from build123d import *

# Parameters (mm, degrees)
SM_BASE_FLANGE_1_DEPTH   = 61.75
SKETCH_3_R               = 25
CUT_EXTRUDE_1_DEPTH      = 4
EXTRUDE_2_DEPTH          = 4
CUT_EXTRUDE_3_DEPTH      = 4
SM_START                 = -122
SM_EDGE_FLANGE_1_DEPTH   = 244
SM_EDGE_FLANGE_1_2_DEPTH = 33
SM_START_2               = 89
SM_EDGE_FLANGE_1_3_DEPTH = 33
SKETCH_44_R              = 3.25
CUT_EXTRUDE_4_DEPTH      = 4
CHAMFER_1_SIZE           = 4


# Read off the part's stored shape, not the designer's step: Ребро-кромка1
# Sheet-metal steps are written as plain solids
with BuildPart() as part:
    # Sketch 1 → Базовая кромка1 (new, symmetric)
    with BuildSketch(Plane.XY):
        with BuildLine():
            Line((-67.211573407, -134), (-53.127605882, 0))
            Line((-53.127605882, 0), (-50.876471404, 21.418113853))
            ThreePointArc((-50.876471404, 21.418113853), (-49.574906248, 23.972579302), (-46.898383823, 25))
            Line((-46.898383823, 25), (46.898383823, 25))
            ThreePointArc((46.898383823, 25), (49.574906248, 23.972579302), (50.876471404, 21.418113853))
            Line((50.876471404, 21.418113853), (53.127605882, 0))
            Line((53.127605882, 0), (67.211573407, -134))
            Line((67.211573407, -134), (71.189660989, -133.581886147))
            Line((71.189660989, -133.581886147), (57.105693463, 0.418113853))
            Line((57.105693463, 0.418113853), (54.854558986, 21.836227706))
            ThreePointArc((54.854558986, 21.836227706), (52.251428674, 26.945158604), (46.898383823, 29))
            Line((46.898383823, 29), (-46.898383823, 29))
            ThreePointArc((-46.898383823, 29), (-52.251428674, 26.945158604), (-54.854558986, 21.836227706))
            Line((-54.854558986, 21.836227706), (-57.105693463, 0.418113853))
            Line((-57.105693463, 0.418113853), (-71.189660989, -133.581886147))
            Line((-71.189660989, -133.581886147), (-67.211573407, -134))
        make_face()
    extrude(amount=SM_BASE_FLANGE_1_DEPTH, both=True)

    # Эскиз3 → Вытянуть1 (cut)
    with BuildSketch(Plane(origin=(0, 29, 0), x_dir=(1, 0, 0), z_dir=(0, 1, 0))):
        with Locations(Location((0, 0, 0), (0, 0, 180))):
            Circle(SKETCH_3_R)
    extrude(amount=-CUT_EXTRUDE_1_DEPTH, mode=Mode.SUBTRACT)

    # Эскиз33 → Вытянуть2 (add)
    with BuildSketch(Plane(origin=(56.525210635, 5.941039037, 0), x_dir=(0, 0, -1), z_dir=(0.9945218953682734, 0.10452846326765315, 0))):
        with BuildLine():
            Line((-62.05448187, 13.177809809), (-121.69551813, -130.808388804))
            ThreePointArc((-121.69551813, -130.808388804), (-121.923141122, -131.558761245), (-122, -132.339122533))
            Line((-122, -132.339122533), (-122, -140.291456461))
            Line((-122, -140.291456461), (-61.75, -140.291456461))
            Line((-61.75, -140.291456461), (-61.75, 14.708543539))
            ThreePointArc((-61.75, 14.708543539), (-61.826858878, 13.928182251), (-62.05448187, 13.177809809))
        make_face()
        with BuildLine():
            Line((122, -132.339122533), (122, -140.291456461))
            Line((122, -140.291456461), (61.75, -140.291456461))
            Line((61.75, -140.291456461), (61.75, 14.708543539))
            ThreePointArc((61.75, 14.708543539), (61.826858878, 13.928182251), (62.05448187, 13.177809809))
            Line((62.05448187, 13.177809809), (121.69551813, -130.808388804))
            ThreePointArc((121.69551813, -130.808388804), (121.923141122, -131.558761245), (122, -132.339122533))
        make_face()
    extrude_2 = extrude(amount=-EXTRUDE_2_DEPTH)

    # Эскиз39 → Вытянуть3 (cut)
    with BuildSketch(Plane(origin=(56.525210635, 5.941039037, 0), x_dir=(0, 0, -1), z_dir=(0.9945218953682734, 0.10452846326765315, 0))):
        with BuildLine():
            Line((25.655356237, -12.291456461), (-25.655356237, -12.291456461))
            ThreePointArc((-25.655356237, -12.291456461), (-27.73044927, -12.871808979), (-29.20339957, -14.444462008))
            Line((-29.20339957, -14.444462008), (-88.548043333, -128.444462008))
            ThreePointArc((-88.548043333, -128.444462008), (-88.885368279, -129.340712892), (-89, -130.291456461))
            Line((-89, -130.291456461), (-89, -140.291456461))
            Line((-89, -140.291456461), (89, -140.291456461))
            Line((89, -140.291456461), (89, -130.291456461))
            ThreePointArc((89, -130.291456461), (88.885368279, -129.340712892), (88.548043333, -128.444462008))
            Line((88.548043333, -128.444462008), (29.20339957, -14.444462008))
            ThreePointArc((29.20339957, -14.444462008), (27.73044927, -12.871808979), (25.655356237, -12.291456461))
        make_face()
    cut_extrude_3 = extrude(amount=-CUT_EXTRUDE_3_DEPTH, mode=Mode.SUBTRACT)

    # Зеркальное отражение1: Вытянуть2, Вытянуть3 across plane
    add(extrude_2.mirror(Plane(origin=(0, 0, 0), x_dir=(0, 0, 1), z_dir=(1, 0, 0))))
    add(cut_extrude_3.mirror(Plane(origin=(0, 0, 0), x_dir=(0, 0, 1), z_dir=(1, 0, 0))), mode=Mode.SUBTRACT)

    # Ребро-кромка1 outline → Ребро-кромка1 (cut)
    with BuildSketch(Plane.XY.offset(SM_START)):
        with BuildLine():
            Line((71.189660989, -133.581886147), (71.116967081, -132.890249808))
            ThreePointArc((71.116967081, -132.890249808), (67.89872427, -130.284168166), (66.414685062, -126.418113853))
            Line((66.414685062, -126.418113853), (67.211573407, -134))
            Line((67.211573407, -134), (71.189660989, -133.581886147))
        make_face()
        with BuildLine():
            ThreePointArc((-66.414685062, -126.418113853), (-67.89872427, -130.284168166), (-71.116967081, -132.890249808))
            Line((-71.116967081, -132.890249808), (-71.189660989, -133.581886147))
            Line((-71.189660989, -133.581886147), (-67.211573407, -134))
            Line((-67.211573407, -134), (-66.414685062, -126.418113853))
        make_face()
    extrude(amount=SM_EDGE_FLANGE_1_DEPTH, mode=Mode.SUBTRACT)

    # Sm Edge Flange 1 2 outline → Sm Edge Flange 1 2 (add)
    with BuildSketch(Plane.XY.offset(SM_START)):
        with BuildLine():
            ThreePointArc((71.116967081, -132.890249808), (72.707566699, -133.407066953), (74.370860225, -133.581886147))
            Line((74.370860225, -133.581886147), (98.769244048, -133.581886147))
            Line((98.769244048, -133.581886147), (98.769244048, -129.581886147))
            Line((98.769244048, -129.581886147), (74.370860225, -129.581886147))
            ThreePointArc((74.370860225, -129.581886147), (71.694337799, -128.554465449), (70.392772643, -126))
            Line((70.392772643, -126), (71.116967081, -132.890249808))
        make_face()
        with BuildLine():
            Line((-98.769244048, -133.581886147), (-74.370860225, -133.581886147))
            ThreePointArc((-74.370860225, -133.581886147), (-72.707566699, -133.407066953), (-71.116967081, -132.890249808))
            Line((-71.116967081, -132.890249808), (-70.392772643, -126))
            ThreePointArc((-70.392772643, -126), (-71.694337799, -128.554465449), (-74.370860225, -129.581886147))
            Line((-74.370860225, -129.581886147), (-98.769244048, -129.581886147))
            Line((-98.769244048, -129.581886147), (-98.769244048, -133.581886147))
        make_face()
    extrude(amount=SM_EDGE_FLANGE_1_2_DEPTH)

    # Sm Edge Flange 1 3 outline → Sm Edge Flange 1 3 (add)
    with BuildSketch(Plane.XY.offset(SM_START_2)):
        with BuildLine():
            ThreePointArc((71.116967081, -132.890249808), (72.707566699, -133.407066953), (74.370860225, -133.581886147))
            Line((74.370860225, -133.581886147), (98.769244048, -133.581886147))
            Line((98.769244048, -133.581886147), (98.769244048, -129.581886147))
            Line((98.769244048, -129.581886147), (74.370860225, -129.581886147))
            ThreePointArc((74.370860225, -129.581886147), (71.694337799, -128.554465449), (70.392772643, -126))
            Line((70.392772643, -126), (71.116967081, -132.890249808))
        make_face()
        with BuildLine():
            Line((-98.769244048, -133.581886147), (-74.370860225, -133.581886147))
            ThreePointArc((-74.370860225, -133.581886147), (-72.707566699, -133.407066953), (-71.116967081, -132.890249808))
            Line((-71.116967081, -132.890249808), (-70.392772643, -126))
            ThreePointArc((-70.392772643, -126), (-71.694337799, -128.554465449), (-74.370860225, -129.581886147))
            Line((-74.370860225, -129.581886147), (-98.769244048, -129.581886147))
            Line((-98.769244048, -129.581886147), (-98.769244048, -133.581886147))
        make_face()
    extrude(amount=SM_EDGE_FLANGE_1_3_DEPTH)

    # Эскиз44 → Вытянуть4 (cut)
    with BuildSketch(Plane(origin=(0, -129.581886147, 0), x_dir=(1, 0, 0), z_dir=(0, 1, 0))):
        with Locations(Location((90, -112.5, 0), (0, 0, 180))):
            Circle(SKETCH_44_R)
        with Locations(Location((90, 112.5, 0), (0, 0, 180))):
            Circle(SKETCH_44_R)
        with Locations(Location((-90, 112.5, 0), (0, 0, 180))):
            Circle(SKETCH_44_R)
        with Locations(Location((-90, -112.5, 0), (0, 0, 180))):
            Circle(SKETCH_44_R)
    extrude(amount=-CUT_EXTRUDE_4_DEPTH, mode=Mode.SUBTRACT)

    # Фаска1
    chamfer_1_edges = [part.edges().sort_by_distance(p)[0] for p in [
        (98.769244048, -131.581886147, 122),
        (98.769244048, -131.581886147, 89),
        (-98.769244048, -131.581886147, 89),
        (-98.769244048, -131.581886147, 122),
        (98.769244048, -131.581886147, -89),
        (98.769244048, -131.581886147, -122),
        (-98.769244048, -131.581886147, -122),
        (-98.769244048, -131.581886147, -89),
    ]]
    chamfer(chamfer_1_edges, length=CHAMFER_1_SIZE)


solid = part.part
Source: CAD feature listing. Evaluate the final solid. Frame: model axes, mm. A direction names the side the tool comes from. Give positions to 0.01 mm unless a question says otherwise; leave off trailing zeros. Write each loop counter-clockwise with the first axis right and the second up, starting at its lowest first coordinate (ties: lowest second). Pieces come first, ordered by that corner, then holes. Notation, with made-up numbers: (-4, 28) -> (32, 28) arc R9 ccw to (32, 35) -> close; hole circle Ø5 at (37, 35.25). An arc over 180 degrees is marked (long way). Write item = value, one per line.
Q1. First-contact query: pin 1 (7 mm diameter, centred on x = 7, y = 26, fed in from +Z); pin 2 (19.5 mm diameter, centred on x = 88, z = 109, fed in from +Y). Flat tips, straight axial feed; report the tip coordinate or a pass-through.
Here are the results:
pin_1 = 61.75
pin_2 = -129.58
Q2. Cut plane A-A on x = 0. Return loops of the section in (y, z).
Here are the results:
outline = (25, -61.75) -> (29, -61.75) -> (29, -25) -> (25, -25) -> close; (25, 25) -> (29, 25) -> (29, 61.75) -> (25, 61.75) -> close
Q3. Cut plane B-B on z = 0. Return loops of the section in (x, y), then the cut area to 3 significant figures.
Here are the results:
outline = (-57.81, -6.28) -> (-53.83, -6.7) -> (-50.88, 21.42) arc R4 cw to (-46.9, 25) -> (-25, 25) -> (-25, 29) -> (-46.9, 29) arc R8 ccw to (-54.85, 21.84) -> close; (25, 25) -> (46.9, 25) arc R4 cw to (50.88, 21.42) -> (53.83, -6.7) -> (57.81, -6.28) -> (54.85, 21.84) arc R8 ccw to (46.9, 29) -> (25, 29) -> close
area = 472 mm²
Q4. Line query: line 1 (Z direction, x = 90, y = -132.65); line 2 (Z direction, x = 0, y = 28.1); line 3 (Y direction, x = 13, z = 42.5). Output: solid intervals per line, ascending. Write a range as from..to.
Here are the results:
line_1 = -122..-115.75, -109.25..-89, 89..109.25, 115.75..122
line_2 = -61.75..-25, 25..61.75
line_3 = 25..29
Q5. Cut plane C-C on x = -90. Return loops of the section in (y, z), then the cut area to 3 significant figures.
Here are the results:
outline = (-133.58, -122) -> (-129.58, -122) -> (-129.58, -115.75) -> (-133.58, -115.75) -> close; (-133.58, -109.25) -> (-129.58, -109.25) -> (-129.58, -89) -> (-133.58, -89) -> close; (-133.58, 89) -> (-129.58, 89) -> (-129.58, 109.25) -> (-133.58, 109.25) -> close; (-133.58, 115.75) -> (-129.58, 115.75) -> (-129.58, 122) -> (-133.58, 122) -> close
area = 212 mm²
Q6. Reachability of faces 1 (the face through (62.12, -66.11, -59.29)), 2 (the face through (80, -131, 89)) from +Z, -Z, +X, -X, +Y, -Y: full face, straight path, thin tool, end or side. Return the list, or none.
Here are the results:
face_1 = +X, -Y
face_2 = +X, -X, -Y
Q7. Cut plane D-D on y = 14.5. Return loops of the section in (x, z), then the cut area to 3 significant figures.
Here are the results:
outline = (-55.63, -63.95) -> (-51.6, -63.77) -> (-51.6, 63.77) -> (-55.63, 63.95) -> close; (51.6, -63.77) -> (55.63, -63.95) -> (55.63, 63.95) -> (51.6, 63.77) -> close
area = 1,030 mm²
Q8. Mould query, pull axis X, two halves, no side actions, for faces 3 (the face through (90.705, -131.554, -115.673)), 4 (the face through (-62.12, -66.11, -59.29)), 5 (the face through (-79, -131, 89)), 6 (the face through (-23.846, 27.028, 7.509)). Classes: +X half, -X half, draft (parallel to the pull), parting line (faces both ways), or undercut.
Here are the results:
face_3 = undercut
face_4 = -X half
face_5 = draft
face_6 = undercut
